Autodesk Inventor part; units mm, degrees
ref_plane "YZ Plane" through (0, 0, 0) normal (1, 0, 0) x (0, 1, 0)
ref_plane "XZ Plane" through (0, 0, 0) normal (0, 1, 0) x (-1, 0, 0)
ref_plane "XY Plane" through (0, 0, 0) normal (0, 0, 1) x (1, 0, 0)
sketch "Skizze4" plane through (0, 0, 0) normal (1, 0, 0) x (0, 1, 0)
  line L0 (-15.675, 9.95) -> (15.675, 9.95)
  line L1 (15.675, 9.95) -> (15.675, -9.95)
  line L2 (15.675, -9.95) -> (-15.675, -9.95)
  line L3 (-15.675, -9.95) -> (-15.675, 9.95)
  line L4 (0, -13.93) -> (0, 13.93) construction
  line L5 (-21.945, 0) -> (21.945, 0) construction
  point P0 (0, 0)
  dimension "d4" = 31.35
  dimension "d5" = 19.9
extrude "Extrusion2" add sketch "Skizze4" along normal blind 12.1
sketch "Skizze5" plane through (0, 0, 0) normal (0, 1, 0) x (-1, 0, 0)
  circle A0 centre (0, 0) radius 2
  dimension "d8" = 4
extrude "Extrusion3" cut sketch "Skizze5" along normal mid plane 20
fillet "Rundung1" radius 2 2 edges at (2, -10, 0) (2, 10, 0)
sketch "Skizze6" plane through (0, 0, 0) normal (-1, 0, 0) x (0, 0, 1)
  line L0 (-6.95, 7.675) -> (-6.95, -12.325) construction
  line L1 (9.95, 15.675) -> (-9.95, 15.675) construction
  line L2 (-9.95, 15.675) -> (-9.95, -15.675) construction
  line L3 (-6.95, 11.675) -> (6.95, 11.675) construction
  line L4 (6.95, 11.675) -> (6.95, -12.325) construction
  line L5 (9.95, -15.675) -> (9.95, 15.675) construction
  point P0 (0, 0)
  dimension "d12" = 4
  dimension "d15" = 4
  dimension "d16" = 24
  dimension "d17" = 3
  dimension "d18" = 24
  dimension "d19" = 3
hole "Bohrung1" at (0, 7.675, -6.95) at (0, 11.675, -6.95) at (0, -12.325, -6.95) at (0, 11.675, 6.95) at (0, -12.325, 6.95) direction (1, 0, 0) diameter 1 depth 2 tip angle 118
sketch "Skizze7" plane through (12.1, 0, 0) normal (1, 0, 0) x (0, 0, -1)
  line L0 (-8.0362, 11.2286) -> (8.4274, 11.2286) construction
  line L1 (8.4274, 11.2286) -> (8.4274, -13.5124) construction
  line L2 (8.4274, -13.5124) -> (-8.0362, -13.5124) construction
  line L3 (-8.0362, -13.5124) -> (-8.0362, 11.2286) construction
  point P0 (0, 0)
equation "\"d19\" = d17"
properties part number "LDD-1000LW" material "Kst - PTFE(white)"
Verification items for the finished model (mm, model axes). A direction names the side the tool comes from. Give positions to 0.01 mm unless a question says otherwise; leave off trailing zeros. Loops run counter-clockwise (first coordinate to the right, second up) from the corner with the lowest first, then second, coordinate; pieces in that order, holes last. Notation, with made-up numbers: (-8, -38.5) - (50, -38.5) arc R25 cw to (50, -21.5) - close; hole circle Ø2 at (26.25, -15.75). An arc over 180 degrees is marked (long way). Write each question's results on one line, items separated by ' | '.
1) Mould release check, pull along Z, two halves, no side actions. Record for faces 1 (the flat face through (6, 0, -9.95)), 2 (the conical face through (2.25, 11.6, -6.91)), 3 (the flat face through (6, 15.675, 0)): pulls with the +Z half, pulls with the -Z half, needs draft (parallel to the pull), parting line crosses it, or undercut.
Solution:
face 1: pulls with the -Z half | face 2: undercut | face 3: needs draft
2) Sectioned sample at A-A on y = -1. Record the boundary of the cut face in (x, z), plus the area to 3 significant figures.
Solution:
outline: (0, -9.95) - (12.1, -9.95) - (12.1, 9.95) - (0, 9.95) - (0, 2) arc R2 cw to (0, -2) - close | area: 235 mm2
3) Tool access check on faces 4 (the cylindrical face through (1.014, -12.747, -6.681)), 5 (the flat face through (0, -0.2, 2.4)). Record the directions out of +Z, -Z, +X, -X, +Y, -Y that give a thin tool (end or side, any length) a straight path to the whole face; none if there is none.
Solution:
face 4: -X | face 5: +Z, -Z, -X, +Y, -Y
4) Material ranges on L1, parallel to Y at x = 1, z = -6.95 (3 decimals); L2, parallel to Y at x = 1.25, z = 6.95 (3 decimals); L3, parallel to Z at x = 1.5, y = 0, recorded low to high. Write a range as from..to.
Solution:
L1: -15.675..-12.825, -11.825..7.175, 8.175..11.175, 12.175..15.675 | L2: -15.675..-12.825, -11.825..11.175, 12.175..15.675 | L3: -9.95..-1.32, 1.32..9.95
